The model under review builds one solid part; all positions refer to its coordinate system, in mm. Face numbers are marked on the shaded views. A direction names the side the tool comes from. Coordinates: 2 decimals unless noted, no trailing zeros. Write each loop counter-clockwise with the first axis right and the second up, starting at its lowest first coordinate (ties: lowest second). Pieces come first, ordered by that corner, then holes.
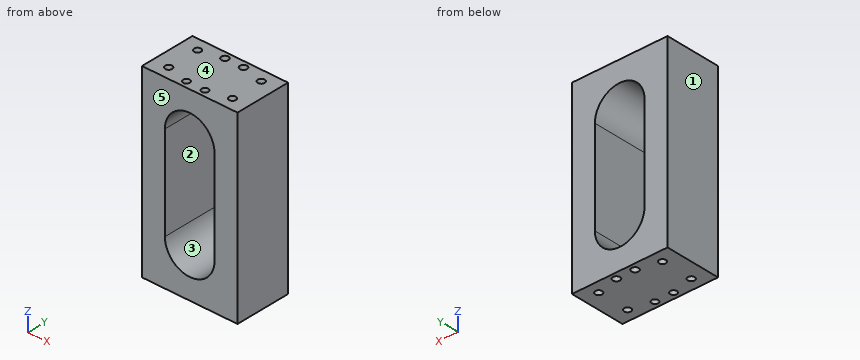
```python
from build123d import *

# Parameters (mm, degrees)
SKETCH_1_W          = 36
SKETCH_1_H          = 21
SKETCH_1_R          = 1.25
SKETCH_1_R_2        = 1.3
SKETCH_1_R_3        = 1.35
EXTRUDE_1_DEPTH     = 70
SKETCH_1_5_R        = 1.3
SKETCH_1_5_R_2      = 1.35
SKETCH_1_5_R_3      = 1.25
CUT_EXTRUDE_1_DEPTH = 4
CUT_EXTRUDE_START   = 70
SKETCH_1_6_R        = 1.35
SKETCH_1_6_R_2      = 1.3
SKETCH_1_6_R_3      = 1.25
CUT_EXTRUDE_2_DEPTH = 4
CUT_EXTRUDE1_DEPTH  = 30


with BuildPart() as part:
    # 스케치1 → 보스-돌출1 (new body)
    with BuildSketch(Plane.XY):
        Rectangle(SKETCH_1_W, SKETCH_1_H)
        with Locations((-3.5, -8)):
            Circle(SKETCH_1_R, mode=Mode.SUBTRACT)
        with Locations((3.5, -8)):
            Circle(SKETCH_1_R, mode=Mode.SUBTRACT)
        with Locations((-12, 6)):
            Circle(SKETCH_1_R_2, mode=Mode.SUBTRACT)
        with Locations((12, 6)):
            Circle(SKETCH_1_R_2, mode=Mode.SUBTRACT)
        with Locations((12, -6)):
            Circle(SKETCH_1_R_2, mode=Mode.SUBTRACT)
        with Locations((-12, -6)):
            Circle(SKETCH_1_R_2, mode=Mode.SUBTRACT)
        with Locations((3.5, 8)):
            Circle(SKETCH_1_R_3, mode=Mode.SUBTRACT)
        with Locations((-3.5, 8)):
            Circle(SKETCH_1_R_3, mode=Mode.SUBTRACT)
        with Locations((12, -6)):
            Circle(SKETCH_1_R_2)
        with Locations((3.5, -8)):
            Circle(SKETCH_1_R)
        with Locations((-3.5, -8)):
            Circle(SKETCH_1_R)
        with Locations((-12, -6)):
            Circle(SKETCH_1_R_2)
        with Locations((-12, 6)):
            Circle(SKETCH_1_R_2)
        with Locations((-3.5, 8)):
            Circle(SKETCH_1_R_3)
        with Locations((3.5, 8)):
            Circle(SKETCH_1_R_3)
        with Locations((12, 6)):
            Circle(SKETCH_1_R_2)
    extrude(amount=EXTRUDE_1_DEPTH)

    # 스케치1<5> → 컷-돌출1 (cut)
    with BuildSketch(Plane.XY):
        with Locations((12, 6)):
            Circle(SKETCH_1_5_R)
        with Locations((3.5, 8)):
            Circle(SKETCH_1_5_R_2)
        with Locations((-3.5, 8)):
            Circle(SKETCH_1_5_R_2)
        with Locations((-12, 6)):
            Circle(SKETCH_1_5_R)
        with Locations((-12, -6)):
            Circle(SKETCH_1_5_R)
        with Locations(Location((-3.5, -8, 0), (0, 0, 180))):
            Circle(SKETCH_1_5_R_3)
        with Locations((3.5, -8)):
            Circle(SKETCH_1_5_R_3)
        with Locations((12, -6)):
            Circle(SKETCH_1_5_R)
    extrude(amount=CUT_EXTRUDE_1_DEPTH, mode=Mode.SUBTRACT)

    # 스케치1<6> → 컷-돌출2 (cut)
    with BuildSketch(Plane.XY.offset(CUT_EXTRUDE_START)):
        with Locations((3.5, 8)):
            Circle(SKETCH_1_6_R)
        with Locations((12, 6)):
            Circle(SKETCH_1_6_R_2)
        with Locations((-3.5, 8)):
            Circle(SKETCH_1_6_R)
        with Locations((-12, 6)):
            Circle(SKETCH_1_6_R_2)
        with Locations((-12, -6)):
            Circle(SKETCH_1_6_R_2)
        with Locations(Location((-3.5, -8, 0), (0, 0, 180))):
            Circle(SKETCH_1_6_R_3)
        with Locations((3.5, -8)):
            Circle(SKETCH_1_6_R_3)
        with Locations((12, -6)):
            Circle(SKETCH_1_6_R_2)
    extrude(amount=-CUT_EXTRUDE_2_DEPTH, mode=Mode.SUBTRACT)

    # Sketch1 → Cut-Extrude1 (cut)
    with BuildSketch(Plane(origin=(0, 10.5, 0), x_dir=(1, 0, 0), z_dir=(0, 1, 0))):
        with BuildLine():
            Line((9.357060489, -17.19326846), (9.357060489, -52.841694339))
            ThreePointArc((9.357060489, -52.841694339), (0, -62.198754828), (-9.357060489, -52.841694339))
            Line((-9.357060489, -52.841694339), (-9.357060489, -17.19326846))
            ThreePointArc((-9.357060489, -17.19326846), (0, -7.836207971), (9.357060489, -17.19326846))
        make_face()
    extrude(amount=-CUT_EXTRUDE1_DEPTH, mode=Mode.SUBTRACT)


solid = part.part
```
Item 1: Take a section at C-C, the plane y = -8. Write out the cut boundary in (x, z).
Solved:
outline: (-18, 0) - (-4.75, 0) - (-4.75, 4) - (-2.25, 4) - (-2.25, 0) - (2.25, 0) - (2.25, 4) - (4.75, 4) - (4.75, 0) - (18, 0) - (18, 70) - (4.75, 70) - (4.75, 66) - (2.25, 66) - (2.25, 70) - (-2.25, 70) - (-2.25, 66) - (-4.75, 66) - (-4.75, 70) - (-18, 70) - close; hole (-9.36, 17.19) arc R9.36 ccw to (9.36, 17.19) - (9.36, 52.84) arc R9.36 ccw to (-9.36, 52.84) - close
Item 2: Take a section at B-B, the plane z = 39. Write out the cut boundary in (x, y), plus the area to 3 significant figures.
Solved:
outline: (-18, -10.5) - (-9.36, -10.5) - (-9.36, 10.5) - (-18, 10.5) - close; (9.36, -10.5) - (18, -10.5) - (18, 10.5) - (9.36, 10.5) - close
area: 363 mm2
Item 3: Mouldability with a two-part tool opening along Z and no side actions: class the marked faces 3, 4 and 5 as pulls with the +Z half, pulls with the -Z half, needs draft (parallel to the pull), parting line crosses it, or undercut.
Solved:
face 3: undercut
face 4: pulls with the +Z half
face 5: needs draft
Item 4: Machinability: for the marked faces 1 and 2, which of the approach directions +Z, -Z, +X, -X, +Y, -Y give a long, thin tool a straight path to every point of the face, cutting with its end or side? Answer none if there is none.
Solved:
face 1: +Z, -Z, -X, +Y, -Y
face 2: +Y, -Y
Item 5: Take a section at A-A, the plane x = 0. Write out the cut boundary in (y, z), plus the area to 3 significant figures.
Solved:
outline: (-10.5, 0) - (10.5, 0) - (10.5, 7.84) - (-10.5, 7.84) - close; (-10.5, 62.2) - (10.5, 62.2) - (10.5, 70) - (-10.5, 70) - close
area: 328 mm2
Item 6: Take a section at D-D, the plane x = -12. Write out the cut boundary in (y, z), plus the area to 3 significant figures.
Solved:
outline: (-10.5, 0) - (-7.3, 0) - (-7.3, 4) - (-4.7, 4) - (-4.7, 0) - (4.7, 0) - (4.7, 4) - (7.3, 4) - (7.3, 0) - (10.5, 0) - (10.5, 70) - (7.3, 70) - (7.3, 66) - (4.7, 66) - (4.7, 70) - (-4.7, 70) - (-4.7, 66) - (-7.3, 66) - (-7.3, 70) - (-10.5, 70) - close
area: 1,430 mm2
Item 7: For pin 1 (0.8 mm diameter, centred on x = -3, y = 8, fed in from -Z); pin 2 (12 mm diameter, centred on x = 1.5, z = 22.5, fed in from -Y); pin 3 (2 mm diameter, centred on x = 3.5, y = -8, fed in from +Z), all flat-tipped, find the tip position at first contact; note any pin that passes through.
Solved:
pin 1: stops at z = 4
pin 2: passes through
pin 3: stops at z = 66
Item 8: To check wall thickness, follow line 1 along Y through (x, z) = (3.5, 69.1); line 2 along Y through (x, z) = (12, 1); line 3 along Z through (x, y) = (0, 8). State the ranges of each line that lie inside material, in increasing order.
Solved:
line 1: y = -10.5 to -9.25, -6.75 to 6.65, 9.35 to 10.5
line 2: y = -10.5 to -7.3, -4.7 to 4.7, 7.3 to 10.5
line 3: z = 0 to 7.84, 62.2 to 70
